The model under review builds one solid part; all positions refer to its coordinate system, in mm. A direction names the side the tool comes from. Round coordinates to 2 decimals unless told otherwise and drop trailing zeros. Order: outer loops, then holes, each group sorted by start corner. A loop starts at its lowest first (then second) coordinate and runs counter-clockwise, first axis right, second up. Notation, with made-up numbers: M 45.5,-19.5 L 63.5,-19.5 A15 cw 63.5,1.5 Z; hole C -20,52 d3. An arc over 180 degrees is marked long. Answer as a JSON object with one key per item and string values. Group by question number.
1) The part is to be moulded in two halves that separate along Y. For faces 1 (the flat face through (-16, 0, 242)), 2 (the cylindrical face through (0, 16, 504)), 3 (the flat face through (-1, -18, 266)), say which applies: +Y half, -Y half, draft (parallel to the pull), parting line (faces both ways), or undercut.
2) Consider section B-B, the plane z = 35.5. Write out the cut boundary in (x, y).
3) For faces 4 (the flat face through (20, 0, 259)), 5 (the flat face through (0, -16, 0)), 6 (the flat face through (23, 0, 2)), list the 3-axis set-ups (+Z, -Z, +X, -X, +Y, -Y) from which the entire face can be reached by the end or side of a thin tool; tool diameter is ignored.
4) Consider section A-A, the plane x = 0. Write out the cut boundary in (y, z), then the cut area to 3 significant figures.
5) Insertion check: pin 1 Ø4 at (x, y) = (13, -12.5) entering from -Z; pin 2 Ø2 at (x, y) = (-18, 3.5) entering from +Z; pin 3 Ø3.5 at (y, z) = (2, 8) entering from +X. Each pin has a flat end and moves straight along its axis. Give the tip position at first contact, or say it passes through.
6) To check wall thickness, follow line 1 (Z direction, x = 0, y = -15); line 2 (X direction, y = 3, z = 62); line 3 (Y direction, x = 7.5, z = 317.5). State the ranges of each line that lie inside material, in increasing order.
```python
from build123d import *

# Parameters (mm, degrees)
SKETCH1_W               = 40
SKETCH1_H               = 36
SKETCH1_W_2             = 32
SKETCH1_H_2             = 28.8
BOSS_EXTRUDE1_DEPTH     = 530
SKETCH2_W               = 50
SKETCH2_H               = 28.8
CUT_EXTRUDE1_DEPTH      = 40
FILLET2_RADIUS          = 20
FILLET2_LENGTH          = 3.6
FILLET3_RADIUS          = 20
FILLET3_LENGTH          = 3.6
CUT_EXTRUDE2_DEPTH      = 532.597592169
CUT_EXTRUDE2_DEPTH_BACK = 532.597592169
SKETCH3_R               = 6
CUT_EXTRUDE3_DEPTH      = 10
SKETCH9_R               = 2.5
BOSS_EXTRUDE2_DEPTH     = 36
FILLET4_R               = 1
FILLET5_R               = 1
CUT_EXTRUDE5_START      = -9
SKETCH12_R              = 5
CUT_EXTRUDE5_DEPTH      = 9
SKETCH14_R              = 5
CUT_EXTRUDE6_DEPTH      = 9


with BuildPart() as part:
    # Sketch1 → Boss-Extrude1 (new body)
    with BuildSketch(Plane.XY):
        Rectangle(SKETCH1_W, SKETCH1_H)
        Rectangle(SKETCH1_W_2, SKETCH1_H_2, mode=Mode.SUBTRACT)
    extrude(amount=BOSS_EXTRUDE1_DEPTH)

    # Sketch2 → Cut-Extrude1 (cut)
    with BuildSketch(Plane.XY.offset(530)):
        Rectangle(SKETCH2_W, SKETCH2_H)
    extrude(amount=-CUT_EXTRUDE1_DEPTH, mode=Mode.SUBTRACT)

    # Fillet2: full round fillet: the end face becomes a half cylinder, R = half its width
    fillet2_face = Plane((0, -16.2, 530), x_dir=(0, -1, 0), z_dir=(0, 0, 1))  # on the end face: x along it, z out of the body
    fillet2_slab = fillet2_face.offset(-FILLET2_RADIUS / 2) * Box(FILLET2_LENGTH, 2 * FILLET2_RADIUS, FILLET2_RADIUS, mode=Mode.PRIVATE)  # the body's end, R deep
    fillet2_round = Plane((0, -16.2, 510), x_dir=(0, 0, 1), z_dir=(0, -1, 0)) * Cylinder(FILLET2_RADIUS, FILLET2_LENGTH, mode=Mode.PRIVATE)  # its axis R under the face
    add(fillet2_slab - fillet2_round, mode=Mode.SUBTRACT)

    # Fillet3: full round fillet: the end face becomes a half cylinder, R = half its width
    fillet3_face = Plane((0, 16.2, 530), x_dir=(0, -1, 0), z_dir=(0, 0, 1))  # on the end face: x along it, z out of the body
    fillet3_slab = fillet3_face.offset(-FILLET3_RADIUS / 2) * Box(FILLET3_LENGTH, 2 * FILLET3_RADIUS, FILLET3_RADIUS, mode=Mode.PRIVATE)  # the body's end, R deep
    fillet3_round = Plane((0, 16.2, 510), x_dir=(0, 0, 1), z_dir=(0, -1, 0)) * Cylinder(FILLET3_RADIUS, FILLET3_LENGTH, mode=Mode.PRIVATE)  # its axis R under the face
    add(fillet3_slab - fillet3_round, mode=Mode.SUBTRACT)

    # Sketch3 → Cut-Extrude2 (cut, two sides: drawn at the far end of the back side and taken through both)
    with BuildSketch(Plane(origin=(0, 18, 0), x_dir=(1, 0, 0), z_dir=(0, 1, 0)).offset(-CUT_EXTRUDE2_DEPTH_BACK)):
        with Locations(Location((0, -510, 0), (0, 0, 270))):
            Circle(SKETCH3_R)
    extrude(amount=CUT_EXTRUDE2_DEPTH + CUT_EXTRUDE2_DEPTH_BACK, mode=Mode.SUBTRACT)

    # Sketch6 → Cut-Extrude3 (cut)
    with BuildSketch(Plane.XZ.offset(18)):
        with BuildLine():
            ThreePointArc((6, 460), (0, 466), (-6, 460))
            Line((-6, 460), (-6, 360))
            ThreePointArc((-6, 360), (0, 354), (6, 360))
            Line((6, 360), (6, 460))
        make_face()
    extrude(amount=-CUT_EXTRUDE3_DEPTH, mode=Mode.SUBTRACT)

    # Sketch9 → Boss-Extrude2 (add)
    with BuildSketch(Plane.XZ.offset(18)):
        with BuildLine():
            Line((20, 14.120693524), (20, 0))
            ThreePointArc((20, 0), (29.330127019, -2.5), (22.5, 4.330127019))
            Line((22.5, 4.330127019), (22.5, 14.120693524))
            Line((22.5, 14.120693524), (20, 14.120693524))
        make_face()
        with Locations(Location((25, 0, 0), (0, 0, 270))):
            Circle(SKETCH9_R, mode=Mode.SUBTRACT)
    extrude(amount=-BOSS_EXTRUDE2_DEPTH)

    # Fillet4
    fillet4_edges = [part.edges().sort_by_distance(p)[0] for p in [
        (22.5, 0, 4.330127019),
    ]]
    fillet(fillet4_edges, radius=FILLET4_R)

    # Fillet5
    fillet5_edges = [part.edges().sort_by_distance(p)[0] for p in [
        (22.5, 0, 14.120693524),
    ]]
    fillet(fillet5_edges, radius=FILLET5_R)

    # Sketch12 → Cut-Extrude5 (cut)
    with BuildSketch(Plane(origin=(0, 18, 0), x_dir=(1, 0, 0), z_dir=(0, 1, 0)).offset(CUT_EXTRUDE5_START)):
        with Locations((25, 0)):
            Circle(SKETCH12_R)
    extrude(amount=CUT_EXTRUDE5_DEPTH, mode=Mode.SUBTRACT)

    # Sketch14 → Cut-Extrude6 (cut)
    with BuildSketch(Plane(origin=(0, -9, 0), x_dir=(-1, 0, 0), z_dir=(0, -1, 0))):
        with Locations((-25, 0)):
            Circle(SKETCH14_R)
    extrude(amount=-CUT_EXTRUDE6_DEPTH, mode=Mode.SUBTRACT)


solid = part.part
```
Results list:
{
 "1": {"face 1": "undercut", "face 2": "draft", "face 3": "-Y half"},
 "2": {"outline": "M -20,-18 L 20,-18 L 20,18 L -20,18 Z; hole M -16,-14.4 L 16,-14.4 L 16,14.4 L -16,14.4 Z"},
 "3": {"face 4": "+Z, +X, +Y, -Y", "face 5": "-Z, -X, +Y, -Y", "face 6": "-Z, +X"},
 "4": {"outline": "M -18,0 L -14.4,0 L -14.4,354 L -18,354 Z; M -18,466 L -14.4,466 L -14.4,504 L -18,504 Z; M -18,516 L -14.4,516 L -14.4,530 L -18,530 Z; M 14.4,0 L 18,0 L 18,504 L 14.4,504 Z; M 14.4,516 L 18,516 L 18,530 L 14.4,530 Z", "area": "3,330 mm^2"},
 "5": {"pin 1": "z = 0", "pin 2": "z = 490", "pin 3": "x = 22.5"},
 "6": {"line 1": "0 to 354, 466 to 504, 516 to 530", "line 2": "-20 to -16, 16 to 20", "line 3": "-18 to -14.4, 14.4 to 18"}
}
